Autodesk Inventor part; units mm, degrees
ref_plane "YZ Plane" through (0, 0, 0) normal (1, 0, 0) x (0, 1, 0)
ref_plane "XZ Plane" through (0, 0, 0) normal (0, 1, 0) x (-1, 0, 0)
ref_plane "XY Plane" through (0, 0, 0) normal (0, 0, 1) x (1, 0, 0)
sketch "Sketch3" plane through (-13.672, 63.246, 0) normal (0, 1, 0) x (1, 0, 0)
  line L0 (10.624, 0) -> (10.624, 152.4)
  line L1 (0, 152.4) -> (10.624, 152.4)
  line L2 (0, 0) -> (0, 152.4)
  line L3 (10.624, 0) -> (0, 0)
  point P0 (13.672, 0)
  point P1 (5.312, 127)
  point P2 (5.312, 152.4)
  point P3 (5.312, 101.6)
  point P4 (5.312, 76.2)
  point P5 (5.312, 50.8)
  point P6 (5.312, 25.4)
  dimension "d28" = 25.4
  dimension "d31" = 25.4
sketch "Sketch1" plane through (0, 0, 0) normal (1, 0, 0) x (0, 1, 0)
  line L0 (0, 0) -> (57.15, 0)
  line L1 (57.15, 0) -> (57.15, -152.4)
  line L2 (57.15, -152.4) -> (0, -152.4)
  line L3 (0, -152.4) -> (0, 0)
  circle A0 centre (28.575, -28.575) radius 14.2875
  circle A1 centre (28.575, -60.325) radius 6.35
  circle A2 centre (28.575, -92.075) radius 6.35
  circle A3 centre (28.575, -123.825) radius 14.2875
  circle A4 centre (50.8, -6.35) radius 2.2479
  circle A5 centre (50.8, -146.05) radius 2.2479
  circle A6 centre (6.35, -146.05) radius 2.2479
  circle A7 centre (6.35, -6.35) radius 2.2479
  line L4 (50.8, -6.35) -> (6.35, -6.35) construction
  line L5 (6.35, -6.35) -> (6.35, -146.05) construction
  line L6 (6.35, -146.05) -> (50.8, -146.05) construction
  line L7 (50.8, -146.05) -> (50.8, -6.35) construction
  line L8 (57.15, 0) -> (69.85, 0)
  line L9 (69.85, 0) -> (69.85, -152.4)
  line L10 (69.85, -152.4) -> (57.15, -152.4)
  line L11 (57.15, -152.4) -> (57.15, 0)
  line L12 (0, -152.4) -> (-12.7, -152.4)
  line L13 (-12.7, -152.4) -> (-12.7, 0)
  line L14 (-12.7, 0) -> (0, 0)
  line L15 (0, 0) -> (0, -152.4)
  line L16 (28.575, -123.825) -> (28.575, -28.575)
  point P0 (28.575, -152.4)
  point P1 (28.575, -6.35)
  point P2 (28.575, 0)
  point P3 (50.8, -76.2)
  point P4 (57.15, -76.2)
  point P5 (57.15, -76.2)
  point P6 (28.575, -76.2)
  dimension "d0" = 57.15
  dimension "d1" = 152.4
  dimension "d2" = 31.75
  dimension "d3" = 31.75
  dimension "d4" = 31.75
  dimension "d6" = 28.575
  dimension "d7" = 12.7
  dimension "d8" = 28.575
  dimension "d11" = 4.4958
  dimension "d12" = 139.7
  dimension "d13" = 44.45
  dimension "d14" = 12.7
  dimension "d15" = 152.4
  dimension "d16" = 12.7
  dimension "d17" = 152.4
extrude "Plate2" add sketch "Sketch1" along normal blind 3.048 contours L0 L1 L2 L3
sketch "Sketch2" plane through (-3.048, 60.198, -152.4) normal (0, 1, 0) x (-1, 0, 0)
  line L0 (0, 152.4) -> (0, 0)
  line L1 (0, 0) -> (10.624, 0)
  line L2 (10.624, 0) -> (10.624, 152.4)
  line L3 (10.624, 152.4) -> (0, 152.4)
edge flange "Flange1" height 16.72 angle 90 thickness 3.048 bend radius 3.048 thickness toward (0, 1, 0) relief tear relief width 3.048 relief depth 1.524 corner gap 3.048 corner form 0 edges at (0, 57.15, -76.2) (0, 0, -76.2) wall of the first edge with corners at (-3.048, 60.198, 0) (-3.048, 60.198, -152.4) (-13.672, 60.198, -152.4) (-13.672, 60.198, 0)
bend "Bend1"
corner "Corner1"
sketch "Sketch4" plane through (-10.624, -3.048, -152.4) normal (-1, 0, 0) x (0, -1, 0)
  line L0 (0, 152.4) -> (0, 0)
  line L1 (0, 0) -> (23.048, 0)
  line L2 (23.048, 0) -> (23.048, 152.4)
  line L3 (23.048, 152.4) -> (0, 152.4)
edge flange "Flange2" height 20 angle 90 thickness 3.048 bend radius 3.048 thickness toward (-1, 0, 0) relief tear relief width 3.048 relief depth 1.524 edges at (-13.672, -6.096, -76.2) wall of the first edge with corners at (-10.624, -3.048, 0) (-10.624, -3.048, -152.4) (-10.624, -26.096, -152.4) (-10.624, -26.096, 0)
bend "Bend2"
corner "Corner2"
sketch "Sketch5" plane through (-10.624, -26.096, 0) normal (1, 0, 0) x (0, 0, -1)
  line L0 (152.4, 16.952) -> (152.4, 0)
  line L1 (0, 0) -> (152.4, 0)
  point P0 (0, 26.096)
  point P1 (127, 10)
  point P2 (101.6, 10)
  point P3 (76.2, 10)
  point P4 (50.8, 10)
  point P5 (25.4, 10)
  dimension "d53" = 25.4
  dimension "d54" = 10
  dimension "d57" = 25.4
hole "Hole2" at (-10.624, -16.096, -127) at (-10.624, -16.096, -101.6) at (-10.624, -16.096, -76.2) at (-10.624, -16.096, -50.8) at (-10.624, -16.096, -25.4) direction (-1, 0, 0) diameter 4.134 end through all
equation "\"d10\" = Thickness"
equation "\"d18\" = BendReliefWidth"
equation "\"d19\" = BendReliefDepth"
equation "\"d20\" = MinimumRemnant"
equation "\"d21\" = TransitionRadius"
equation "\"d24\" = BendRadius"
equation "\"d25\" = CornerReliefSize"
equation "\"d26\" = GapSize"
equation "\"d27\" = JacobiRadiusSize"
equation "\"d43\" = BendReliefWidth"
equation "\"d44\" = BendReliefDepth"
equation "\"d45\" = MinimumRemnant"
equation "\"d46\" = TransitionRadius"
equation "\"d49\" = BendRadius"
equation "\"d50\" = CornerReliefSize"
equation "\"d51\" = GapSize"
equation "\"d52\" = JacobiRadiusSize"
equation "\"BendRadius\" = Thickness"
equation "\"BendReliefWidth\" = Thickness"
equation "\"BendReliefDepth\" = 0.5 * Thickness"
equation "\"CornerReliefSize\" = 4 * Thickness"
equation "\"MinimumRemnant\" = 2 * Thickness"
equation "\"TransitionRadius\" = BendRadius"
equation "\"JacobiRadiusSize\" = BendRadius"
equation "\"GapSize\" = Thickness"
properties part number "CH-1-01-GearboxHousingMotorSide" material "Steel, Alloy"
Here's how the part is built. I have some questions about the finished solid (model axes, mm). A direction names the side the tool comes from. Coordinates: 2 decimals unless noted, no trailing zeros. Loops run counter-clockwise (first coordinate to the right, second up) from the corner with the lowest first, then second, coordinate; pieces in that order, holes last. Notation, with made-up numbers: (20.5, 4) -> (72.5, 4) arc R3 cw to (72.5, 9) -> close; hole circle Ø1 at (39.25, 51.25). An arc over 180 degrees is marked (long way). Return JSON: item names as keys, results as strings.
1) If we section it at D-D, the plane y = 37.5: Write out the boundary of the cut face in (x, z).
Results below:
{"outline": "(0, -152.4) -> (3.05, -152.4) -> (3.05, -134.98) -> (0, -134.98) -> close; (0, -112.67) -> (3.05, -112.67) -> (3.05, -39.73) -> (0, -39.73) -> close; (0, -17.42) -> (3.05, -17.42) -> (3.05, 0) -> (0, 0) -> close"}
2) If we section it at B-B, the plane z = -146.05: Write out the boundary of the cut face in (x, y).
Results below:
{"outline": "(-13.67, -26.1) -> (-10.62, -26.1) -> (-10.62, -9.14) arc R3.05 cw to (-7.58, -6.1) -> (-3.05, -6.1) arc R6.1 ccw to (3.05, 0) -> (3.05, 4.1) -> (0, 4.1) -> (0, 0) arc R3.05 cw to (-3.05, -3.05) -> (-7.58, -3.05) arc R6.1 ccw to (-13.67, -9.14) -> close; (-13.67, 60.2) -> (-3.05, 60.2) arc R3.05 cw to (0, 57.15) -> (0, 53.05) -> (3.05, 53.05) -> (3.05, 57.15) arc R6.1 ccw to (-3.05, 63.25) -> (-13.67, 63.25) -> close; (0, 8.6) -> (3.05, 8.6) -> (3.05, 48.55) -> (0, 48.55) -> close"}
3) If we section it at C-C, the plane z = -50.8: Write out the boundary of the cut face in (x, y), then the cut area to 3 significant figures.
Results below:
{"outline": "(-13.67, -26.1) -> (-10.62, -26.1) -> (-10.62, -18.16) -> (-13.67, -18.16) -> close; (-13.67, -14.03) -> (-10.62, -14.03) -> (-10.62, -9.14) arc R3.05 cw to (-7.58, -6.1) -> (-3.05, -6.1) arc R6.1 ccw to (3.05, 0) -> (3.05, 57.15) arc R6.1 ccw to (-3.05, 63.25) -> (-13.67, 63.25) -> (-13.67, 60.2) -> (-3.05, 60.2) arc R3.05 cw to (0, 57.15) -> (0, 0) arc R3.05 cw to (-3.05, -3.05) -> (-7.58, -3.05) arc R6.1 ccw to (-13.67, -9.14) -> close", "area": "325 mm²"}
4) If we section it at A-A, the plane y = 6.35: Write out the boundary of the cut face in (x, z), then the cut area to 3 significant figures.
Results below:
{"outline": "(0, -152.4) -> (3.05, -152.4) -> (3.05, -148.3) -> (0, -148.3) -> close; (0, -143.8) -> (3.05, -143.8) -> (3.05, -8.6) -> (0, -8.6) -> close; (0, -4.1) -> (3.05, -4.1) -> (3.05, 0) -> (0, 0) -> close", "area": "437 mm²"}
5) Thinking about a two-plate mould opening in Y: for faces 4 (the face through (1.21, 61.51, -77.27)), 5 (the face through (-13.672, -20, -77)), 6 (the face through (-0.92, -2.18, -75.13)), which applies, +Y half, -Y half, draft (parallel to the pull), parting line (faces both ways), or undercut?
Results below:
{"face 4": "+Y half", "face 5": "draft", "face 6": "undercut"}
6) I need wall thicknesses on line 1 (Y direction, x = -6, z = -85); line 2 (Y direction, x = -11.8, z = -25.4); line 3 (Y direction, x = -12.1, z = -50.8). Which ranges of each line are inside material? Lowest first, please. Write a range as from..to.
Results below:
{"line 1": "-6.1..-3.05, 60.2..63.25", "line 2": "-26.1..-18.16, -14.03..-4.75, 60.2..63.25", "line 3": "-26.1..-18.16, -14.03..-5.06, 60.2..63.25"}
7) Will these pins go through, and if not, where does the flat tip stop? pin 1 (3.5 mm diameter, centred on y = -16.096, z = -76.2, fed in from +X); pin 2 (6 mm diameter, centred on y = -5, z = -17.5, fed in from -X); pin 3 (5 mm diameter, centred on x = -7, z = -122, fed in from -Y); pin 4 (6 mm diameter, centred on y = 33.5, z = -113, fed in from -X).
Results below:
{"pin 1": "through", "pin 2": "x = -13.56", "pin 3": "y = -6.78", "pin 4": "x = 0"}
8) For faces 1 (the face through (0, 28, -75)), 2 (the face through (-5, -6.096, -75)), 3 (the face through (3.048, 28, -75)), which set-ups out of +Z, -Z, +X, -X, +Y, -Y let a thin tool reach every point of the face, with its end or its side?
Results below:
{"face 1": "+Z, -Z, -X", "face 2": "+Z, -Z, +X, -Y", "face 3": "+Z, -Z, +X, +Y, -Y"}
